Check sheet for the modelled part. Datum: model origin and axes. Units: mm. Give positions to 0.01 mm unless a question says otherwise; leave off trailing zeros. Order: outer loops, then holes, each group sorted by start corner. A loop starts at its lowest first (then second) coordinate and runs counter-clockwise, first axis right, second up.
```python
from build123d import *

# Parameters (mm, degrees)
BOSS_EXTRUDE1_DEPTH = 4
SKETCH2_W           = 429.121378383
SKETCH2_H           = 424.720133477
CUT_EXTRUDE1_DEPTH  = 10


with BuildPart() as part:
    # Sketch1 → Boss-Extrude1 (new body)
    with BuildSketch(Plane.XY):
        Polygon((88.868642116, -197.391367321), (-88.868642116, -197.391367321), (-88.868642116, -217.665581629), (-129.454428553, -258.251368066), (-150.131357884, -258.251368066), (-150.131357884, -476.251366576), (-129.454428553, -476.251366576), (-88.868642116, -516.837153014), (-88.868642116, -537.111367321), (88.868642116, -537.111367321), (88.868642116, -516.837153014), (129.454428553, -476.251366576), (150.131357884, -476.251366576), (150.131357884, -258.251368066), (129.454428553, -258.251368066), (88.868642116, -217.665581629), align=None)
    extrude(amount=BOSS_EXTRUDE1_DEPTH)

    # Sketch2 → Cut-Extrude1 (cut)
    with BuildSketch(Plane.XY.offset(4)):
        with Locations((25.344127001, -373.74675893)):
            Rectangle(SKETCH2_W, SKETCH2_H)
        Polygon((-83.394427808, -212.191367321), (83.394427808, -212.191367321), (135.331357884, -264.128297397), (135.331357884, -470.374437245), (83.394427808, -522.311367321), (-83.394427808, -522.311367321), (-135.331357884, -470.374437245), (-135.331357884, -264.128297397), align=None, mode=Mode.SUBTRACT)
    extrude(amount=-CUT_EXTRUDE1_DEPTH, mode=Mode.SUBTRACT)


solid = part.part
```
(1) Material ranges on L1, parallel to Y at x = -106.5, z = 0.9; L2, parallel to X at y = -482, z = 3.85; L3, parallel to X at y = -499.5, z = 1.6, recorded low to high.
Response values:
L1: y = -499.21 to -235.3
L2: x = -123.71 to 123.71
L3: x = -106.21 to 106.21
(2) Cross-section at C-C on y = -485. Enter the section's corners in (x, z).
Response values:
outline: (-120.71, 0) - (120.71, 0) - (120.71, 4) - (-120.71, 4) - close
(3) Cross-section at B-B on x = -104. Enter the section's corners in (y, z).
Response values:
outline: (-501.71, 0) - (-232.8, 0) - (-232.8, 4) - (-501.71, 4) - close
(4) Cross-section at A-A on z = 3. Enter the section's corners in (x, y).
Response values:
outline: (-135.33, -470.37) - (-83.39, -522.31) - (83.39, -522.31) - (135.33, -470.37) - (135.33, -264.13) - (83.39, -212.19) - (-83.39, -212.19) - (-135.33, -264.13) - close
